from build123d import *

# Parameters (mm, degrees)
SKETCH_1_W      = 410
SKETCH_1_H      = 70
SKETCH_1_R      = 3
SKETCH_1_R_2    = 6.5
SKETCH_1_R_3    = 1.5
EXTRUDE_1_DEPTH = 3


with BuildPart() as part:
    # 草图1 → 凸台-拉伸1 (new body)
    with BuildSketch(Plane.XY):
        with Locations((205, 35)):
            Rectangle(SKETCH_1_W, SKETCH_1_H)
        with Locations((10, 60)):
            Circle(SKETCH_1_R, mode=Mode.SUBTRACT)
        with Locations((50, 60)):
            Circle(SKETCH_1_R, mode=Mode.SUBTRACT)
        with Locations((80, 60)):
            Circle(SKETCH_1_R, mode=Mode.SUBTRACT)
        with Locations((120, 60)):
            Circle(SKETCH_1_R, mode=Mode.SUBTRACT)
        with Locations((150, 60)):
            Circle(SKETCH_1_R, mode=Mode.SUBTRACT)
        with Locations((190, 60)):
            Circle(SKETCH_1_R, mode=Mode.SUBTRACT)
        with Locations((220, 60)):
            Circle(SKETCH_1_R, mode=Mode.SUBTRACT)
        with Locations((260, 60)):
            Circle(SKETCH_1_R, mode=Mode.SUBTRACT)
        with Locations((290, 60)):
            Circle(SKETCH_1_R, mode=Mode.SUBTRACT)
        with Locations((330, 60)):
            Circle(SKETCH_1_R, mode=Mode.SUBTRACT)
        with Locations((360, 60)):
            Circle(SKETCH_1_R, mode=Mode.SUBTRACT)
        with Locations((400, 60)):
            Circle(SKETCH_1_R, mode=Mode.SUBTRACT)
        with Locations((66.32685934, 26.157789308)):
            Circle(SKETCH_1_R_2, mode=Mode.SUBTRACT)
        with Locations((136.32685934, 26.157789308)):
            Circle(SKETCH_1_R_2, mode=Mode.SUBTRACT)
        with Locations((206.32685934, 26.157789308)):
            Circle(SKETCH_1_R_2, mode=Mode.SUBTRACT)
        with Locations((276.32685934, 26.157789308)):
            Circle(SKETCH_1_R_2, mode=Mode.SUBTRACT)
        with Locations((346.32685934, 26.157789308)):
            Circle(SKETCH_1_R_2, mode=Mode.SUBTRACT)
        with Locations((81.82685934, 33.157789308)):
            Circle(SKETCH_1_R_3, mode=Mode.SUBTRACT)
        with Locations((74.07685934, 19.73439555)):
            Circle(SKETCH_1_R_3, mode=Mode.SUBTRACT)
        with Locations((58.57685934, 19.73439555)):
            Circle(SKETCH_1_R_3, mode=Mode.SUBTRACT)
        with Locations((50.82685934, 33.157789308)):
            Circle(SKETCH_1_R_3, mode=Mode.SUBTRACT)
        with Locations((58.57685934, 46.581183067)):
            Circle(SKETCH_1_R_3, mode=Mode.SUBTRACT)
        with Locations((74.07685934, 46.581183067)):
            Circle(SKETCH_1_R_3, mode=Mode.SUBTRACT)
        with Locations((128.57685934, 46.581183067)):
            Circle(SKETCH_1_R_3, mode=Mode.SUBTRACT)
        with Locations((120.82685934, 33.157789308)):
            Circle(SKETCH_1_R_3, mode=Mode.SUBTRACT)
        with Locations((128.57685934, 19.73439555)):
            Circle(SKETCH_1_R_3, mode=Mode.SUBTRACT)
        with Locations((144.07685934, 19.73439555)):
            Circle(SKETCH_1_R_3, mode=Mode.SUBTRACT)
        with Locations((144.07685934, 46.581183067)):
            Circle(SKETCH_1_R_3, mode=Mode.SUBTRACT)
        with Locations((151.82685934, 33.157789308)):
            Circle(SKETCH_1_R_3, mode=Mode.SUBTRACT)
        with Locations((198.57685934, 46.581183067)):
            Circle(SKETCH_1_R_3, mode=Mode.SUBTRACT)
        with Locations((190.82685934, 33.157789308)):
            Circle(SKETCH_1_R_3, mode=Mode.SUBTRACT)
        with Locations((198.57685934, 19.73439555)):
            Circle(SKETCH_1_R_3, mode=Mode.SUBTRACT)
        with Locations((214.07685934, 19.73439555)):
            Circle(SKETCH_1_R_3, mode=Mode.SUBTRACT)
        with Locations((214.07685934, 46.581183067)):
            Circle(SKETCH_1_R_3, mode=Mode.SUBTRACT)
        with Locations((221.82685934, 33.157789308)):
            Circle(SKETCH_1_R_3, mode=Mode.SUBTRACT)
        with Locations((268.57685934, 46.581183067)):
            Circle(SKETCH_1_R_3, mode=Mode.SUBTRACT)
        with Locations((260.82685934, 33.157789308)):
            Circle(SKETCH_1_R_3, mode=Mode.SUBTRACT)
        with Locations((268.57685934, 19.73439555)):
            Circle(SKETCH_1_R_3, mode=Mode.SUBTRACT)
        with Locations((284.07685934, 19.73439555)):
            Circle(SKETCH_1_R_3, mode=Mode.SUBTRACT)
        with Locations((284.07685934, 46.581183067)):
            Circle(SKETCH_1_R_3, mode=Mode.SUBTRACT)
        with Locations((291.82685934, 33.157789308)):
            Circle(SKETCH_1_R_3, mode=Mode.SUBTRACT)
        with Locations((338.57685934, 46.581183067)):
            Circle(SKETCH_1_R_3, mode=Mode.SUBTRACT)
        with Locations((330.82685934, 33.157789308)):
            Circle(SKETCH_1_R_3, mode=Mode.SUBTRACT)
        with Locations((338.57685934, 19.73439555)):
            Circle(SKETCH_1_R_3, mode=Mode.SUBTRACT)
        with Locations((354.07685934, 19.73439555)):
            Circle(SKETCH_1_R_3, mode=Mode.SUBTRACT)
        with Locations((354.07685934, 46.581183067)):
            Circle(SKETCH_1_R_3, mode=Mode.SUBTRACT)
        with Locations((361.82685934, 33.157789308)):
            Circle(SKETCH_1_R_3, mode=Mode.SUBTRACT)
        with Locations((325, 44)):
            Circle(SKETCH_1_R_3, mode=Mode.SUBTRACT)
        with Locations((321, 19)):
            Circle(SKETCH_1_R_3, mode=Mode.SUBTRACT)
        with Locations((255, 44)):
            Circle(SKETCH_1_R_3, mode=Mode.SUBTRACT)
        with Locations((251, 19)):
            Circle(SKETCH_1_R_3, mode=Mode.SUBTRACT)
        with Locations((185, 44)):
            Circle(SKETCH_1_R_3, mode=Mode.SUBTRACT)
        with Locations((181, 19)):
            Circle(SKETCH_1_R_3, mode=Mode.SUBTRACT)
        with Locations((115, 44)):
            Circle(SKETCH_1_R_3, mode=Mode.SUBTRACT)
        with Locations((111, 19)):
            Circle(SKETCH_1_R_3, mode=Mode.SUBTRACT)
        with Locations((45, 44)):
            Circle(SKETCH_1_R_3, mode=Mode.SUBTRACT)
        with Locations((41, 19)):
            Circle(SKETCH_1_R_3, mode=Mode.SUBTRACT)
        with Locations((400, 10)):
            Circle(SKETCH_1_R, mode=Mode.SUBTRACT)
        with Locations((10, 10)):
            Circle(SKETCH_1_R, mode=Mode.SUBTRACT)
        with Locations((10, 35)):
            Circle(SKETCH_1_R, mode=Mode.SUBTRACT)
        with Locations((400, 35)):
            Circle(SKETCH_1_R, mode=Mode.SUBTRACT)
    extrude(amount=EXTRUDE_1_DEPTH)


solid = part.part
The listing builds one solid part. Answer for the finished solid, in the listing's coordinates (mm). Coordinates: 2 decimals unless noted, no trailing zeros. Write each loop counter-clockwise with the first axis right and the second up, starting at its lowest first coordinate (ties: lowest second). Pieces come first, ordered by that corner, then holes. Notation, with made-up numbers: M 35,-9.5 L 73,-9.5 A29 ccw 73,29.5 Z; hole C 47.25,26.5 d7. An arc over 180 degrees is marked long. Put each result on its own line as item: value. Start each with the question number.
1. A flat-ended cylindrical pin translates along its axis: P1, Ø5, axis at x = 198.58, y = 19.73, coming from the -Z side. Find the tip coordinate at first contact, or state that the pin passes through.
2. For a pull along Y with two mould halves and no side action, classify faces 1 (the flat face through (202, 35, 3)), 2 (the cylindrical face through (142.527, 28.11, 1.479)) as pulls with the +Y half, pulls with the -Y half, needs draft (parallel to the pull), parting line crosses it, or undercut.
3. A cutting plane is placed at B-B on x = 207. Write down the section's boundary in (y, z).
4. Consider line 1 (X direction, y = 9.5, z = 1.1); line 2 (Y direction, x = 321, z = 1.1); line 3 (Y direction, x = 277, z = 0.35). Determine where each line is inside the solid, lowest interval first. Write a range as from..to.
5. A cutting plane is placed at C-C on z = 1.25. Count the separate pieces of the cut face and the enclosed holes in it, then the cut area to 3 significant figures.
6. A cutting plane is placed at A-A on x = 65. Write down the section's boundary in (y, z), then the cut area to 3 significant figures.
Resolved:
1. P1: stops at z = 0
2. face 1: needs draft
2. face 2: undercut
3. outline: M 0,0 L 19.69,0 L 19.69,3 L 0,3 Z; M 32.62,0 L 70,0 L 70,3 L 32.62,3 Z
4. line 1: x = 0..7.04, 12.96..397.04, 402.96..410
4. line 2: y = 0..17.5, 20.5..70
4. line 3: y = 0..19.69, 32.62..70
5. separate pieces: 1
5. enclosed holes: 61
5. area: 27,300 mm2
6. outline: M 0,0 L 19.79,0 L 19.79,3 L 0,3 Z; M 32.52,0 L 70,0 L 70,3 L 32.52,3 Z
6. area: 172 mm2
